The drawing under review shows one solid part. Ordinate dimensions are in mm from its lowest x, y, z. Round coordinates to 2 decimals unless told otherwise and drop trailing zeros. Order: outer loops, then holes, each group sorted by start corner. A loop starts at its lowest first (then second) coordinate and runs counter-clockwise, first axis right, second up. Notation, with made-up numbers: M 74,-22.75 L 115,-22.75 A26 ccw 115,-5.75 Z; hole C 38,28 d9. An arc over 180 degrees is marked long. Answer as a JSON object with one key per item and string values.
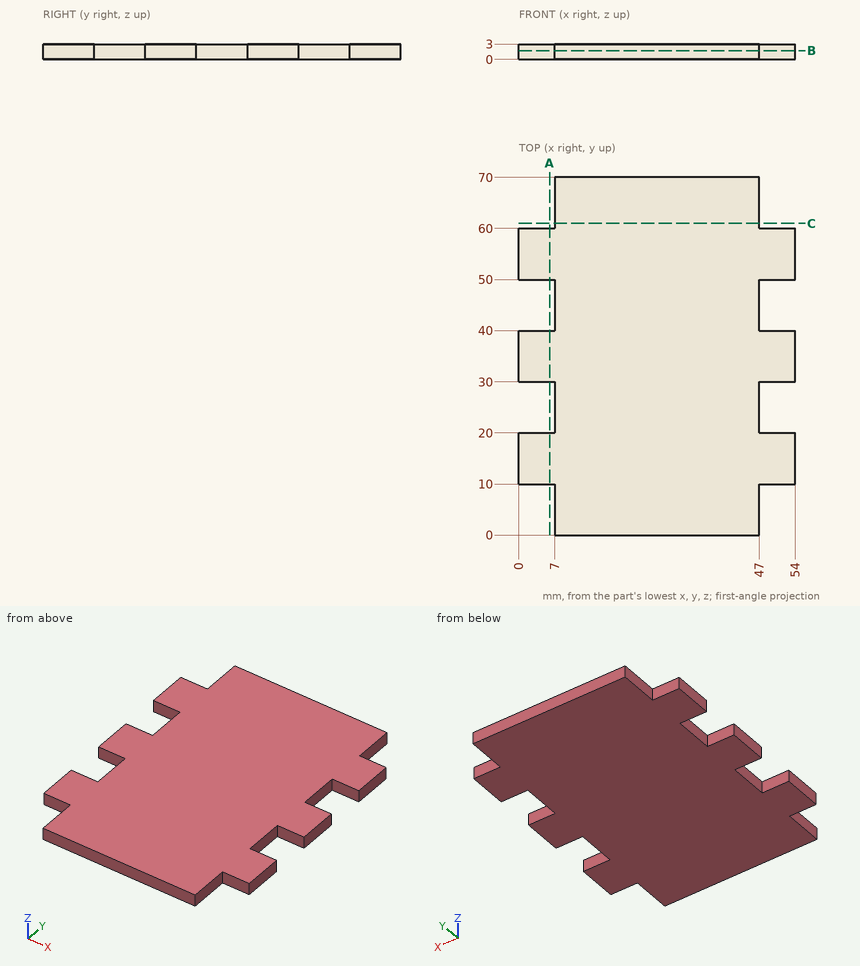
1) Add section B-B on z = 1.7. State the section outline as (x, y) points.
Geometry check:
{"outline": "M 0,10 L 7,10 L 7,0 L 47,0 L 47,10 L 54,10 L 54,20 L 47,20 L 47,30 L 54,30 L 54,40 L 47,40 L 47,50 L 54,50 L 54,60 L 47,60 L 47,70 L 7,70 L 7,60 L 0,60 L 0,50 L 7,50 L 7,40 L 0,40 L 0,30 L 7,30 L 7,20 L 0,20 Z"}
2) Add section A-A on x = 6. State the section outline as (y, z) points.
Geometry check:
{"outline": "M 10,0 L 20,0 L 20,3 L 10,3 Z; M 30,0 L 40,0 L 40,3 L 30,3 Z; M 50,0 L 60,0 L 60,3 L 50,3 Z"}
3) Add section C-C on y = 61. State the section outline as (x, z) points, and give its area (3 significant figures).
Geometry check:
{"outline": "M 7,0 L 47,0 L 47,3 L 7,3 Z", "area": "120 mm²"}
4) For L1, parallel to Y at x = 4.5, z = 0.45; L2, parallel to X at y = 20.5, z = 2.2, list the stretches that pass through material, from the lowest coordinate up.
Geometry check:
{"L1": "y = 10 to 20, 30 to 40, 50 to 60", "L2": "x = 7 to 47"}
5) Insertion check: P1, Ø1.5, axis at y = 23.5, z = 2, coming from the -X side; P2, Ø1.5, axis at x = 4, z = 2, coming from the -Y side; P3, Ø1.5, axis at y = 26, z = 1.5, coming from the +X side. Each pin has a flat end and moves straight along its axis. Give the tip position at first contact, or say it passes through.
Geometry check:
{"P1": "stops at x = 7", "P2": "stops at y = 10", "P3": "stops at x = 47"}
